Geometry: final body of the model. Coordinates: model frame, mm. Face numbers are marked on the shaded views. A direction names the side the tool comes from. Give positions to 0.01 mm unless a question says otherwise; leave off trailing zeros. Order: outer loops, then holes, each group sorted by start corner. A loop starts at its lowest first (then second) coordinate and runs counter-clockwise, first axis right, second up. Notation, with made-up numbers: M -40,3 L 4,3 A17 cw 4,11 Z; hole C 50,0 d4. An arc over 180 degrees is marked long. Use CSV: the item, a comma, the result in double quotes.
```python
from build123d import *

# Parameters (mm, degrees)
F0_R     = 35
F0_R_2   = 3.2880949383
F0_R_3   = 24.5
F0_R_4   = 22
F0_R_5   = 6.6571375288
F0_R_6   = 1.75
F1_DEPTH = 5
F2_DEPTH = 25
F3_DEPTH = 3


with BuildPart() as f1:
    # F0 (on Top) → F1 (new body)
    with BuildSketch(Plane.XY):
        Circle(F0_R)
        with Locations((-17.5033363634, -24.0912757185)):
            Circle(F0_R_2, mode=Mode.SUBTRACT)
        with Locations((-6.1912888152, -29.1277237765)):
            Circle(F0_R_2, mode=Mode.SUBTRACT)
        with Locations((-25.7888980415, -14.8892272264)):
            Circle(F0_R_2, mode=Mode.SUBTRACT)
        with Locations((-29.6153249635, -3.1126960824)):
            Circle(F0_R_2, mode=Mode.SUBTRACT)
        with Locations((6.1912888152, -29.1277237765)):
            Circle(F0_R_2, mode=Mode.SUBTRACT)
        with Locations((17.5033363634, -24.0912757185)):
            Circle(F0_R_2, mode=Mode.SUBTRACT)
        with Locations((25.7888980415, -14.8892272264)):
            Circle(F0_R_2, mode=Mode.SUBTRACT)
        with Locations((29.6153249635, -3.1126960824)):
            Circle(F0_R_2, mode=Mode.SUBTRACT)
        with Locations((-28.3209931525, 9.2020484921)):
            Circle(F0_R_2, mode=Mode.SUBTRACT)
        with Locations((-22.1297043373, 19.9256752844)):
            Circle(F0_R_2, mode=Mode.SUBTRACT)
        with Locations((-12.1119886001, 27.2039718009)):
            Circle(F0_R_2, mode=Mode.SUBTRACT)
        Circle(F0_R_3, mode=Mode.SUBTRACT)
        with Locations((28.3209931525, 9.2020484921)):
            Circle(F0_R_2, mode=Mode.SUBTRACT)
        with Locations((0, 29.7784544528)):
            Circle(F0_R_2, mode=Mode.SUBTRACT)
        with Locations((12.1119886001, 27.2039718009)):
            Circle(F0_R_2, mode=Mode.SUBTRACT)
        with Locations((22.1297043373, 19.9256752844)):
            Circle(F0_R_2, mode=Mode.SUBTRACT)
        Circle(F0_R_3)
        Circle(F0_R_4, mode=Mode.SUBTRACT)
        Circle(F0_R_4)
        with Locations((0, -11.8328090757)):
            Circle(F0_R_5, mode=Mode.SUBTRACT)
        with Locations((-11.8328090757, 0)):
            Circle(F0_R_5, mode=Mode.SUBTRACT)
        Circle(F0_R_6, mode=Mode.SUBTRACT)
        with Locations((11.8328090757, 0)):
            Circle(F0_R_5, mode=Mode.SUBTRACT)
        with Locations((0, 11.8328090757)):
            Circle(F0_R_5, mode=Mode.SUBTRACT)
    extrude(amount=F1_DEPTH)

    # F0 (on Top) → F2 (join)
    with BuildSketch(Plane.XY):
        Circle(F0_R_3)
        Circle(F0_R_4, mode=Mode.SUBTRACT)
    extrude(amount=F2_DEPTH)

    # F0 (on Top) → F3 (join)
    with BuildSketch(Plane.XY):
        Circle(F0_R)
        with Locations((-17.5033363634, -24.0912757185)):
            Circle(F0_R_2, mode=Mode.SUBTRACT)
        with Locations((-6.1912888152, -29.1277237765)):
            Circle(F0_R_2, mode=Mode.SUBTRACT)
        with Locations((-25.7888980415, -14.8892272264)):
            Circle(F0_R_2, mode=Mode.SUBTRACT)
        with Locations((-29.6153249635, -3.1126960824)):
            Circle(F0_R_2, mode=Mode.SUBTRACT)
        with Locations((6.1912888152, -29.1277237765)):
            Circle(F0_R_2, mode=Mode.SUBTRACT)
        with Locations((17.5033363634, -24.0912757185)):
            Circle(F0_R_2, mode=Mode.SUBTRACT)
        with Locations((25.7888980415, -14.8892272264)):
            Circle(F0_R_2, mode=Mode.SUBTRACT)
        with Locations((29.6153249635, -3.1126960824)):
            Circle(F0_R_2, mode=Mode.SUBTRACT)
        with Locations((-28.3209931525, 9.2020484921)):
            Circle(F0_R_2, mode=Mode.SUBTRACT)
        with Locations((-22.1297043373, 19.9256752844)):
            Circle(F0_R_2, mode=Mode.SUBTRACT)
        with Locations((-12.1119886001, 27.2039718009)):
            Circle(F0_R_2, mode=Mode.SUBTRACT)
        Circle(F0_R_3, mode=Mode.SUBTRACT)
        with Locations((28.3209931525, 9.2020484921)):
            Circle(F0_R_2, mode=Mode.SUBTRACT)
        with Locations((0, 29.7784544528)):
            Circle(F0_R_2, mode=Mode.SUBTRACT)
        with Locations((12.1119886001, 27.2039718009)):
            Circle(F0_R_2, mode=Mode.SUBTRACT)
        with Locations((22.1297043373, 19.9256752844)):
            Circle(F0_R_2, mode=Mode.SUBTRACT)
    extrude(amount=F3_DEPTH)


solid = f1.part
```
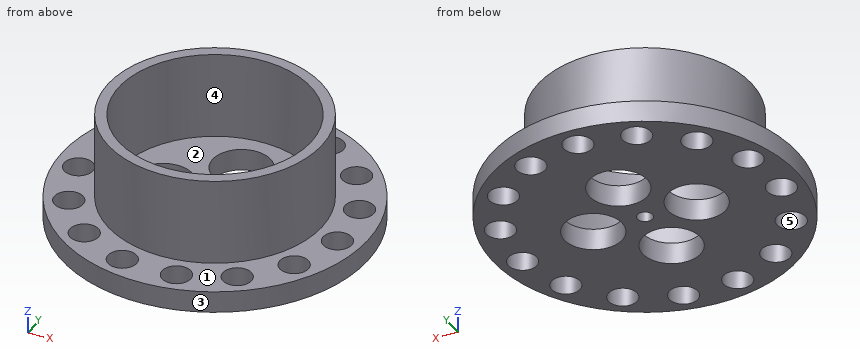
1. Section C-C, the plane x = 30. Return the cut outline in (y, z).
Answer:
outline,"M -18.03,0 L -6.38,0 L -6.38,5 L -18.03,5 Z; M 0.15,0 L 6.37,0 L 6.37,5 L 0.15,5 Z; M 12.03,0 L 18.03,0 L 18.03,5 L 12.03,5 Z"
2. Pull-direction query (Y, two-part tool) for the marked faces 1, 2 and 3; classes: +Y half, -Y half, draft (parallel to the pull), parting line (faces both ways), or undercut.
Answer:
face 1,"draft"
face 2,"undercut"
face 3,"parting line"
3. Section B-B, the plane y = -23. Return the cut outline in (x, z).
Answer:
outline,"M -26.38,0 L -20.61,0 L -20.61,5 L -26.38,5 Z; M -14.4,0 L 14.4,0 L 14.4,5 L 8.44,5 L 8.44,25 L -8.44,25 L -8.44,5 L -14.4,5 Z; M 20.61,0 L 26.38,0 L 26.38,5 L 20.61,5 Z"
4. Section A-A, the plane x = 0. Return the cut outline in (y, z).
Answer:
outline,"M -35,0 L -18.49,0 L -18.49,5 L -22,5 L -22,25 L -24.5,25 L -24.5,5 L -35,5 Z; M -5.18,0 L -1.75,0 L -1.75,5 L -5.18,5 Z; M 1.75,0 L 5.18,0 L 5.18,5 L 1.75,5 Z; M 18.49,0 L 26.49,0 L 26.49,5 L 24.5,5 L 24.5,25 L 22,25 L 22,5 L 18.49,5 Z; M 33.07,0 L 35,0 L 35,5 L 33.07,5 Z"
5. Pin query (flat end, axial travel): pin 1 Ø12 at (x, y) = (-11.83, 0) entering from -Z; pin 2 Ø4 at (x, z) = (-1, 12) entering from -Y; pin 3 Ø12 at (x, z) = (-8.5, 2.5) entering from -Y; pin 4 Ø10 at (x, z) = (-21, 13.5) entering from +Y. Return the tip coordinate at first contact, or that it passes through.
Answer:
pin 1,"through"
pin 2,"y = -24.5"
pin 3,"y = -34.91"
pin 4,"y = 18.55"
6. Section D-D, the plane z = 23.75. Return the cut outline in (x, y).
Answer:
outline,"C 0,0 d49; hole C 0,0 d44"
7. Line query: line 1 (Y direction, x = 0, z = 3.7); line 2 (Y direction, x = 0.5, z = 7.5); line 3 (Y direction, x = -6, z = 1.75). Output: solid intervals per line, ascending.
Answer:
line 1,"-35 to -18.49, -5.18 to -1.75, 1.75 to 5.18, 18.49 to 26.49, 33.07 to 35"
line 2,"-24.49 to -21.99, 21.99 to 24.49"
line 3,"-34.48 to -32.41, -25.85 to -14.72, -8.95 to -3.21, 3.21 to 8.95, 14.72 to 34.48"
8. Reachability of the marked faces 4 and 5 from +Z, -Z, +X, -X, +Y, -Y: full face, straight path, thin tool, end or side. Return the list, or none.
Answer:
face 4,"+Z"
face 5,"+Z, -Z"
